```python
from build123d import *

# Parameters (mm, degrees)
SKETCH_F_W                   = 449
SKETCH_F_H                   = 79
SKETCH_F_R                   = 1.361667817
ESTRUSIONE_ESTRUSIONE1_DEPTH = 3
SKETCH1_R                    = 1.7
EXTRUDE1_DEPTH               = 456.906788719


with BuildPart() as part:
    # Sketch f → Estrusione-Estrusione1 (new body)
    with BuildSketch(Plane.XY):
        with Locations((224.5, 39.5)):
            Rectangle(SKETCH_F_W, SKETCH_F_H)
        with Locations((11.5, 67.5)):
            Circle(SKETCH_F_R, mode=Mode.SUBTRACT)
        with Locations(Location((437.5, 67.5, 0), (0, 0, 180))):
            Circle(SKETCH_F_R, mode=Mode.SUBTRACT)
        with Locations(Location((11.5, 11.5, 0), (0, 0, 180))):
            Circle(SKETCH_F_R, mode=Mode.SUBTRACT)
        with Locations((437.5, 11.5)):
            Circle(SKETCH_F_R, mode=Mode.SUBTRACT)
    extrude(amount=ESTRUSIONE_ESTRUSIONE1_DEPTH)

    # Sketch1 → Extrude1 (cut, through all)
    with BuildSketch(Plane(origin=(0, 0, 0), x_dir=(-1, 0, 0), z_dir=(0, 0, -1))):
        with Locations((-413.061242298, 39.505506417)):
            Circle(SKETCH1_R)
        with Locations((-357.061242298, 39.505506417)):
            Circle(SKETCH1_R)
        with BuildLine():
            Line((-364.0746338, 54.394920259), (-406.0746338, 54.394920259))
            ThreePointArc((-406.0746338, 54.394920259), (-408.903060925, 53.223347384), (-410.0746338, 50.394920259))
            Line((-410.0746338, 50.394920259), (-410.0746338, 28.394920259))
            ThreePointArc((-410.0746338, 28.394920259), (-408.903060925, 25.566493134), (-406.0746338, 24.394920259))
            Line((-406.0746338, 24.394920259), (-364.0746338, 24.394920259))
            ThreePointArc((-364.0746338, 24.394920259), (-361.246206675, 25.566493134), (-360.0746338, 28.394920259))
            Line((-360.0746338, 28.394920259), (-360.0746338, 50.394920259))
            ThreePointArc((-360.0746338, 50.394920259), (-361.246206675, 53.223347384), (-364.0746338, 54.394920259))
        make_face()
    extrude(amount=-EXTRUDE1_DEPTH, mode=Mode.SUBTRACT)


solid = part.part
```
CAD build for the part. Positions are in the model's coordinates, mm. Coordinates: 2 decimals unless noted, no trailing zeros. Order: outer loops, then holes, each group sorted by start corner. A loop starts at its lowest first (then second) coordinate and runs counter-clockwise, first axis right, second up. Notation, with made-up numbers: M 45.25,-19.5 L 52.25,-19.5 A12 cw 52.25,-1.5 Z; hole C 54.5,-9 d4. An arc over 180 degrees is marked long. Answer as CSV lines item,"result".
1) Cut at A-A (z = 0.7). List the corners of the cut face in (x, y), then the cut area to 3 significant figures.
Verdict:
outline,"M 0,0 L 449,0 L 449,79 L 0,79 Z; hole C 11.5,11.5 d2.72; hole C 11.5,67.5 d2.72; hole C 357.06,39.51 d3.4; hole M 360.07,28.39 A4 ccw 364.07,24.39 L 406.07,24.39 A4 ccw 410.07,28.39 L 410.07,50.39 A4 ccw 406.07,54.39 L 364.07,54.39 A4 ccw 360.07,50.39 Z; hole C 413.06,39.51 d3.4; hole C 437.5,11.5 d2.72; hole C 437.5,67.5 d2.72"
area,"33,900 mm2"
2) Drill centre lines: L1, parallel to Y at x = 437.5, z = 2.45; L2, parallel to X at y = 67.5, z = 2; L3, parallel to Y at x = 394.5, z = 1. Where is each one in solid material? Low to high. Write a range as from..to.
Verdict:
L1,"0..10.14, 12.86..66.14, 68.86..79"
L2,"0..10.14, 12.86..436.14, 438.86..449"
L3,"0..24.39, 54.39..79"
3) Flat gauge pin, fed straight in: P1, Ø4.5, axis at x = 11.5, y = 67.5, coming from the -Z side. Where does the tip first touch, or does it go through?
Verdict:
P1,"z = 0"
